Source: CAD feature listing. Evaluate the final solid. Frame: model axes, mm. A direction names the side the tool comes from. Give positions to 0.01 mm unless a question says otherwise; leave off trailing zeros. Order: outer loops, then holes, each group sorted by start corner. A loop starts at its lowest first (then second) coordinate and runs counter-clockwise, first axis right, second up.
from build123d import *

# Parameters (mm, degrees)
F0_W     = 3.2
F0_H     = 20.5
F1_DEPTH = 2.8
F2_R     = 0.85
F3_DEPTH = 20
F4_R     = 1
F5_DEPTH = 1.7
F6_R     = 1.5
F7_DEPTH = 1


with BuildPart() as f1:
    # F0 (on Top) → F1 (new body)
    with BuildSketch(Plane.XY):
        with Locations((1.6, 10.25)):
            Rectangle(F0_W, F0_H)
    extrude(amount=F1_DEPTH)

    # F2 (on face) → F3 (cut)
    with BuildSketch(Plane(origin=(0, 20.5, 0), x_dir=(-1, 0, 0), z_dir=(0, 1, 0))):
        with Locations((-1.6, 1.1)):
            Circle(F2_R)
    extrude(amount=-F3_DEPTH, mode=Mode.SUBTRACT)

    # F4 (on face) → F5 (cut)
    with BuildSketch(Plane.XY.offset(2.8)):
        with Locations((1.6, 1.5)):
            Circle(F4_R)
    extrude(amount=-F5_DEPTH, mode=Mode.SUBTRACT)

    # F6 (on face) → F7 (join)
    with BuildSketch(Plane.XY.offset(2.8)):
        with Locations((1.6, 10.25)):
            Circle(F6_R)
    extrude(amount=F7_DEPTH)


solid = f1.part
(1) Access query for faces 1 (the flat face through (2, 0, 1)), 2 (the cylindrical face through (2.29, 8.92, 3.29)). Directions: +Z, -Z, +X, -X, +Y, -Y. A direction counts if a zero-diameter tool reaches every point of the face in a straight line with its end or side. Return the directions, or none.
(2) Section A-A, the plane y = 10.25. Return loops of the section in (x, z).
(3) Pin query (flat end, axial travel): pin 1 Ø0.5 at (x, z) = (1.5, 1) entering from +Y; pin 2 Ø1 at (x, y) = (2, 7.5) entering from +Z. Return the tip coordinate at first contact, or that it passes through.
(4) Section D-D, the plane y = 5.75. Return loops of the section in (x, z), plus the area to 3 significant figures.
(5) Line query: line 1 along Z through (x, y) = (1.65, 13.5); line 2 along X through (y, z) = (7.25, 1.1); line 3 along X through (y, z) = (1.5, 2.35). Output: solid intervals per line, ascending.
(6) Section C-C, the plane y = 1.5. Return loops of the section in (x, z), plus the area to 3 significant figures.
(7) Section B-B, the plane x = 2.2. Return loops of the section in (y, z), plus the area to 3 significant figures.
(8) Draft query along X for faces 3 (the flat face through (2, 0.5, 1)), 4 (the flat face through (3.2, 10, 1)), 5 (the flat face through (0, 10, 1)), 6 (the flat face through (2, 13, 2.8)). Return one class per face: +X half, -X half, draft (parallel to the pull), parting line (faces both ways), or undercut.
Checks:
1. face 1: +Z, -Z, +X, -X, -Y
1. face 2: +Z
2. outline: (0, 0) - (3.2, 0) - (3.2, 2.8) - (3.1, 2.8) - (3.1, 3.8) - (0.1, 3.8) - (0.1, 2.8) - (0, 2.8) - close; hole circle Ø1.7 at (1.6, 1.1)
3. pin 1: stops at y = 0.5
3. pin 2: stops at z = 2.8
4. outline: (0, 0) - (3.2, 0) - (3.2, 2.8) - (0, 2.8) - close; hole circle Ø1.7 at (1.6, 1.1)
4. area: 6.69 mm2
5. line 1: z = 0 to 0.25, 1.95 to 2.8
5. line 2: x = 0 to 0.75, 2.45 to 3.2
5. line 3: x = 0 to 0.6, 2.6 to 3.2
6. outline: (0, 0) - (3.2, 0) - (3.2, 2.8) - (2.6, 2.8) - (2.6, 1.1) - (2.45, 1.1) arc R0.85 cw to (0.75, 1.1) - (0.6, 1.1) - (0.6, 2.8) - (0, 2.8) - close
6. area: 4.43 mm2
7. outline: (0, 0) - (20.5, 0) - (20.5, 0.5) - (0.5, 0.5) - (0.5, 1.7) - (0.7, 1.7) - (0.7, 2.8) - (0, 2.8) - close; (2.3, 1.7) - (20.5, 1.7) - (20.5, 2.8) - (11.62, 2.8) - (11.62, 3.8) - (8.88, 3.8) - (8.88, 2.8) - (2.3, 2.8) - close
7. area: 34.3 mm2
8. face 3: undercut
8. face 4: +X half
8. face 5: -X half
8. face 6: draft
